from build123d import *

# Parameters (mm, degrees)
BOSS_EXTRUDE1_DEPTH     = 2
BOSS_EXTRUDE2_DEPTH     = 4
CUT_EXTRUDE1_DEPTH      = 39.9548816
CUT_EXTRUDE1_DEPTH_BACK = 39.9548816
CHAMFER1_SIZE           = 0.5


with BuildPart() as part:
    # Sketch2 → Boss-Extrude1 (new body)
    with BuildSketch(Plane.XY):
        with BuildLine():
            Line((-26.081641102, -23.253213977), (-23.253213977, -26.081641102))
            ThreePointArc((-23.253213977, -26.081641102), (-21.793308907, -27.057118483), (-20.071233462, -27.399660586))
            Line((-20.071233462, -27.399660586), (-12.899660586, -27.399660586))
            ThreePointArc((-12.899660586, -27.399660586), (-9.717680071, -26.081641102), (-8.399660586, -22.899660586))
            Line((-8.399660586, -22.899660586), (-8.399660586, -12.899660586))
            ThreePointArc((-8.399660586, -12.899660586), (-9.717680071, -9.717680071), (-12.899660586, -8.399660586))
            Line((-12.899660586, -8.399660586), (-22.899660586, -8.399660586))
            ThreePointArc((-22.899660586, -8.399660586), (-26.081641102, -9.717680071), (-27.399660586, -12.899660586))
            Line((-27.399660586, -12.899660586), (-27.399660586, -20.071233462))
            ThreePointArc((-27.399660586, -20.071233462), (-27.057118483, -21.793308907), (-26.081641102, -23.253213977))
        make_face()
    extrude(amount=BOSS_EXTRUDE1_DEPTH)

    # Sketch1 → Boss-Extrude2 (add)
    with BuildSketch(Plane.XY):
        with BuildLine():
            Line((-12.899660586, -10.949660586), (-22.899660586, -10.949660586))
            ThreePointArc((-22.899660586, -10.949660586), (-24.27851881, -11.520802363), (-24.849660586, -12.899660586))
            Line((-24.849660586, -12.899660586), (-24.849660586, -20.071233462))
            ThreePointArc((-24.849660586, -20.071233462), (-24.701225675, -20.817466155), (-24.27851881, -21.450091685))
            Line((-24.27851881, -21.450091685), (-21.450091685, -24.27851881))
            ThreePointArc((-21.450091685, -24.27851881), (-20.817466155, -24.701225675), (-20.071233462, -24.849660586))
            Line((-20.071233462, -24.849660586), (-12.899660586, -24.849660586))
            ThreePointArc((-12.899660586, -24.849660586), (-11.520802363, -24.27851881), (-10.949660586, -22.899660586))
            Line((-10.949660586, -22.899660586), (-10.949660586, -12.899660586))
            ThreePointArc((-10.949660586, -12.899660586), (-11.520802363, -11.520802363), (-12.899660586, -10.949660586))
        make_face()
    extrude(amount=-BOSS_EXTRUDE2_DEPTH)

    # Sketch3 → Cut-Extrude1 (cut, two sides: drawn at the far end of the back side and taken through both)
    with BuildSketch(Plane.XY.offset(-CUT_EXTRUDE1_DEPTH_BACK)):
        Polygon((-21.995634526, -13.803686646), (-13.493013972, -13.493013972), (-13.803686646, -21.995634526), (-21.706864564, -21.706864564), align=None)
    extrude(amount=CUT_EXTRUDE1_DEPTH + CUT_EXTRUDE1_DEPTH_BACK, mode=Mode.SUBTRACT)

    # Chamfer1
    chamfer1_edges = [part.edges().sort_by_distance(p)[0] for p in [
        (-11.520802363, -11.520802363, -4),
        (-10.949660586, -17.899660586, -4),
        (-11.520802363, -24.27851881, -4),
        (-16.485447024, -24.849660586, -4),
        (-20.817466155, -24.701225675, -4),
        (-22.864305247, -22.864305247, -4),
        (-24.701225675, -20.817466155, -4),
        (-24.849660586, -16.485447024, -4),
        (-24.27851881, -11.520802363, -4),
        (-17.899660586, -10.949660586, -4),
        (-21.851249545, -17.755275605, -4),
        (-17.755275605, -21.851249545, -4),
        (-13.648350309, -17.744324249, -4),
        (-17.744324249, -13.648350309, -4),
    ]]
    chamfer(chamfer1_edges, length=CHAMFER1_SIZE)


solid = part.part
Design review of the part built by this model. Coordinates are the model's own, in mm. A direction names the side the tool comes from. Round coordinates to 2 decimals unless told otherwise and drop trailing zeros. Loops run counter-clockwise (first coordinate to the right, second up) from the corner with the lowest first, then second, coordinate; pieces in that order, holes last. Notation, with made-up numbers: (35, -0.5) - (90, -0.5) arc R15 cw to (90, 25.5) - close; hole circle Ø9 at (5.5, 40.25). An arc over 180 degrees is marked (long way). One line per item, written item: value. Start each with the question number.
1) Consider section C-C on y = -16.5. Give the boundary of the cut face in (x, z).
2) Draft analysis for pull direction X (two halves, no side actions). For faces 5 (the flat face through (-21.85, -17.81, -0.79)), 6 (the flat face through (-24.85, -16, -2)), 7 (the conical face through (-11.791, -24.033, -3.865)), state which applies: +X half, -X half, draft (parallel to the pull), parting line (faces both ways), or undercut.
3) Consider section A-A on z = -1.5. Give the boundary of the cut face in (x, y), then the cut area to 3 significant figures.
4) Consider section B-B on x = -18.5. Give the boundary of the cut face in (y, z).
5) Insertion check: pin 1 Ø1 at (x, z) = (-15, -1) entering from -Y; pin 2 Ø1.8 at (x, z) = (-17, -1.5) entering from +Y; pin 3 Ø3 at (y, z) = (-25, -0.5) entering from +X; pin 4 Ø1.5 at (x, z) = (-19, -0.5) entering from -Y. Each pin has a flat end and moves straight along its axis. Give the tip position at first contact, or say it passes through.
6) To check wall thickness, follow L1, parallel to Z at x = -8.75, y = -21.75; L2, parallel to X at y = -17.25, z = -2.5; L3, parallel to Y at x = -21, z = 1.5. State the ranges of each line that lie inside material, in increasing order. Write a range as from..to.
7) Consider section D-D on z = 1.5. Give the boundary of the cut face in (x, y).
8) For faces 1 (the cylindrical face through (-11.506, -11.536, -1.726)), 2 (the flat face through (-17, -24.85, -2)), 3 (the flat face through (-13.646, -17.685, -0.788)), 4 (the flat face through (-22.884, -22.845, -1.726)), list the 3-axis set-ups (+Z, -Z, +X, -X, +Y, -Y) from which the entire face can be reached by the end or side of a thin tool; tool diameter is ignored.
Reported:
1. outline: (-27.4, 0) - (-24.85, 0) - (-24.85, -3.5) - (-24.35, -4) - (-22.4, -4) - (-21.9, -3.5) - (-21.9, 2) - (-27.4, 2) - close; (-13.6, -3.5) - (-13.1, -4) - (-11.45, -4) - (-10.95, -3.5) - (-10.95, 0) - (-8.4, 0) - (-8.4, 2) - (-13.6, 2) - close
2. face 5: undercut
2. face 6: -X half
2. face 7: +X half
3. outline: (-24.85, -20.07) arc R1.95 ccw to (-24.28, -21.45) - (-21.45, -24.28) arc R1.95 ccw to (-20.07, -24.85) - (-12.9, -24.85) arc R1.95 ccw to (-10.95, -22.9) - (-10.95, -12.9) arc R1.95 ccw to (-12.9, -10.95) - (-22.9, -10.95) arc R1.95 ccw to (-24.85, -12.9) - close; hole (-22, -13.8) - (-21.71, -21.71) - (-13.8, -22) - (-13.49, -13.49) - close
3. area: 115 mm^2
4. outline: (-27.4, 0) - (-24.85, 0) - (-24.85, -3.5) - (-24.35, -4) - (-22.32, -4) - (-21.82, -3.5) - (-21.82, 2) - (-27.4, 2) - close; (-13.68, -3.5) - (-13.18, -4) - (-11.45, -4) - (-10.95, -3.5) - (-10.95, 0) - (-8.4, 0) - (-8.4, 2) - (-13.68, 2) - close
5. pin 1: stops at y = -24.85
5. pin 2: stops at y = -10.95
5. pin 3: stops at x = -8.45
5. pin 4: stops at y = -27.4
6. L1: z = 0..2
6. L2: x = -24.85..-21.87, -13.63..-10.95
6. L3: y = -27.3..-21.73, -13.77..-8.4
7. outline: (-27.4, -20.07) arc R4.5 ccw to (-26.08, -23.25) - (-23.25, -26.08) arc R4.5 ccw to (-20.07, -27.4) - (-12.9, -27.4) arc R4.5 ccw to (-8.4, -22.9) - (-8.4, -12.9) arc R4.5 ccw to (-12.9, -8.4) - (-22.9, -8.4) arc R4.5 ccw to (-27.4, -12.9) - close; hole (-22, -13.8) - (-21.71, -21.71) - (-13.8, -22) - (-13.49, -13.49) - close
8. face 1: -Z, +X, +Y
8. face 2: -Z, +X, -X, -Y
8. face 3: +Z, -Z
8. face 4: -Z, -X, -Y
